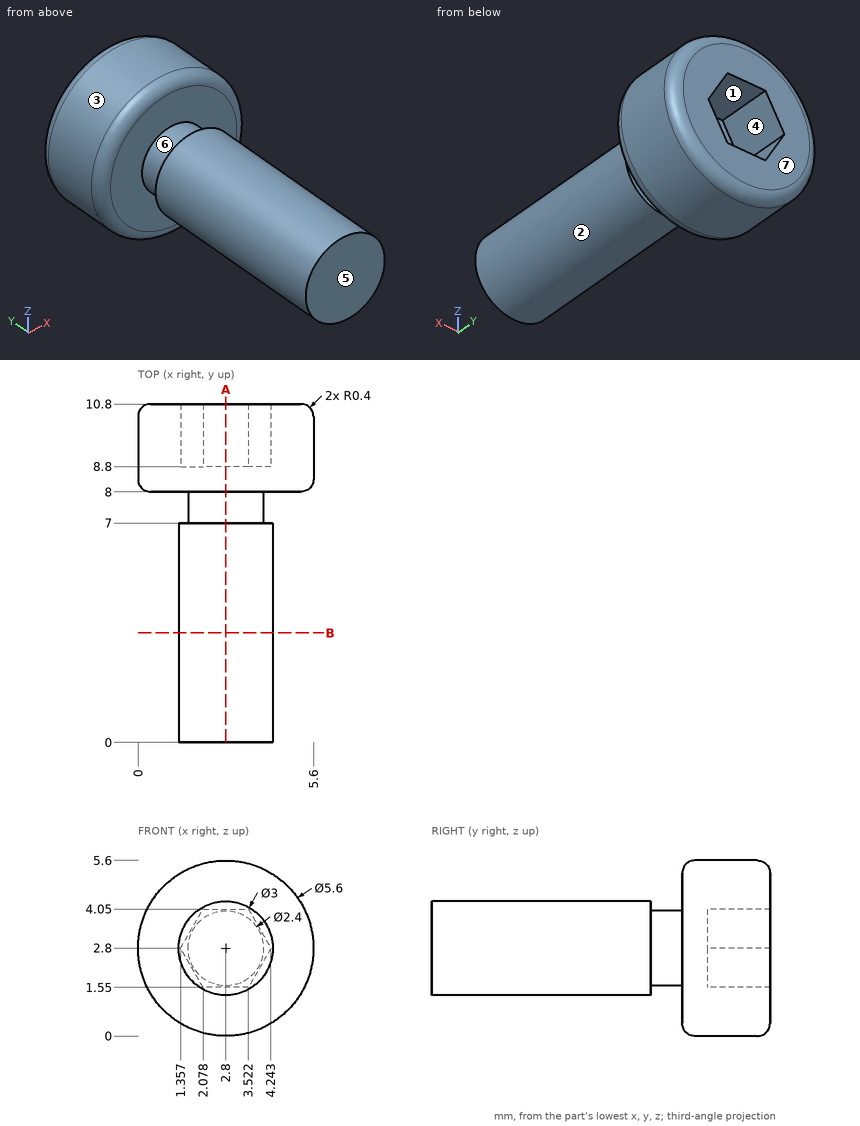
For this review, use the dimensioned drawing (mm, ordinates from the lowest corner) and the shaded views. A direction names the side the tool comes from. Round coordinates to 2 decimals unless told otherwise and drop trailing zeros. Order: outer loops, then holes, each group sorted by start corner. A loop starts at its lowest first (then second) coordinate and runs counter-clockwise, first axis right, second up.
1) Consider section A-A (x = 2.8). State the section outline as (y, z) points.
The answers:
outline: (0, 1.3) - (7, 1.3) - (7, 1.6) - (8, 1.6) - (8, 0.4) arc R0.4 ccw to (8.4, 0) - (10.4, 0) arc R0.4 ccw to (10.8, 0.4) - (10.8, 1.55) - (8.8, 1.55) - (8.8, 4.05) - (10.8, 4.05) - (10.8, 5.2) arc R0.4 ccw to (10.4, 5.6) - (8.4, 5.6) arc R0.4 ccw to (8, 5.2) - (8, 4) - (7, 4) - (7, 4.3) - (0, 4.3) - close
2) Machinability: for the marked faces 1, 2 and 3, which of the approach directions +Z, -Z, +X, -X, +Y, -Y give a long, thin tool a straight path to every point of the face, cutting with its end or side? Answer none if there is none.
The answers:
face 1: +Y
face 2: -Y
face 3: +Y, -Y
3) Clearance check with flat-ended pins moving along their axes: pin 1 Ø1.5 at (y, z) = (8.5, 1) entering from +X (1 decimal); pin 2 Ø3 at (y, z) = (1.5, 4) entering from -X; pin 3 Ø3 at (x, y) = (3.5, 2) entering from -Z. State where each tip first meets the part, or that it passes through.
The answers:
pin 1: stops at x = 5.4
pin 2: stops at x = 1.3
pin 3: stops at z = 1.3
4) Consider section B-B (y = 3.5). State the section outline as (x, z) points.
The answers:
outline: circle Ø3 at (2.8, 2.8)
5) For L1, parallel to Y at x = 3.4, z = 4; L2, parallel to Y at x = 3.15, z = 4.15; L3, parallel to Y at x = 3.1, z = 0.5, list the stretches that pass through material, from the lowest coordinate up.
The answers:
L1: y = 0 to 7, 8 to 8.8
L2: y = 0 to 7, 8 to 10.8
L3: y = 8 to 10.8
6) Draft analysis for pull direction Y (two halves, no side actions). For the marked faces 4, 5, 6 and 7, state which applies: released by +Y, released by -Y, zero draft, split by the parting line, or undercut.
The answers:
face 4: zero draft
face 5: released by -Y
face 6: undercut
face 7: released by +Y
